Could you check a few things on this drawing? It's one solid part, dimensions in mm from its lowest x, y, z. Round coordinates to 2 decimals unless told otherwise and drop trailing zeros. Write each loop counter-clockwise with the first axis right and the second up, starting at its lowest first coordinate (ties: lowest second). Pieces come first, ordered by that corner, then holes. Notation, with made-up numbers: (36, 42) - (68, 42) arc R20 cw to (68, 67) - close; hole circle Ø2 at (42.5, 0.5). An arc over 180 degrees is marked (long way). Use one line per item in the form item = value. Start each with the question number.
1. Will these pins go through, and if not, where does the flat tip stop? pin 1 (8 mm diameter, centred on x = 4, y = 40, fed in from +Z); pin 2 (6 mm diameter, centred on x = 12.7, y = 31.19, fed in from -Z); pin 3 (5.5 mm diameter, centred on x = 12.7, y = 12.7, fed in from -Z) (1 decimal).
2. I want a section at B-B, the plane y = 12.7. List the corners of the cut face in (x, z) for me (1 decimal).
3. I want a section at A-A, the plane z = 10. List the corners of the cut face in (x, y) for me (1 decimal).
4. We'd pull the mould along Y, two halves only. Please class the marked faces 1, 2, 3 and 4: +Y half, -Y half, draft (parallel to the pull), parting line (faces both ways), or undercut.
5. I want a section at D-D, the plane x = 20.5. List the corners of the cut face in (y, z) for me (1 decimal).
6. If I drill on line 1 along Y through (x, z) = (2, 7.75) (1 decimal); line 2 along Y through (x, z) = (19.25, 4.75) (1 decimal); line 3 along Y through (x, z) = (16.75, 4.75) (1 decimal), over which ranges is the centre line in solid material (lowest first)?
7. I want a section at C-C, the plane y = 40.5. List the corners of the cut face in (x, z) for me (1 decimal).
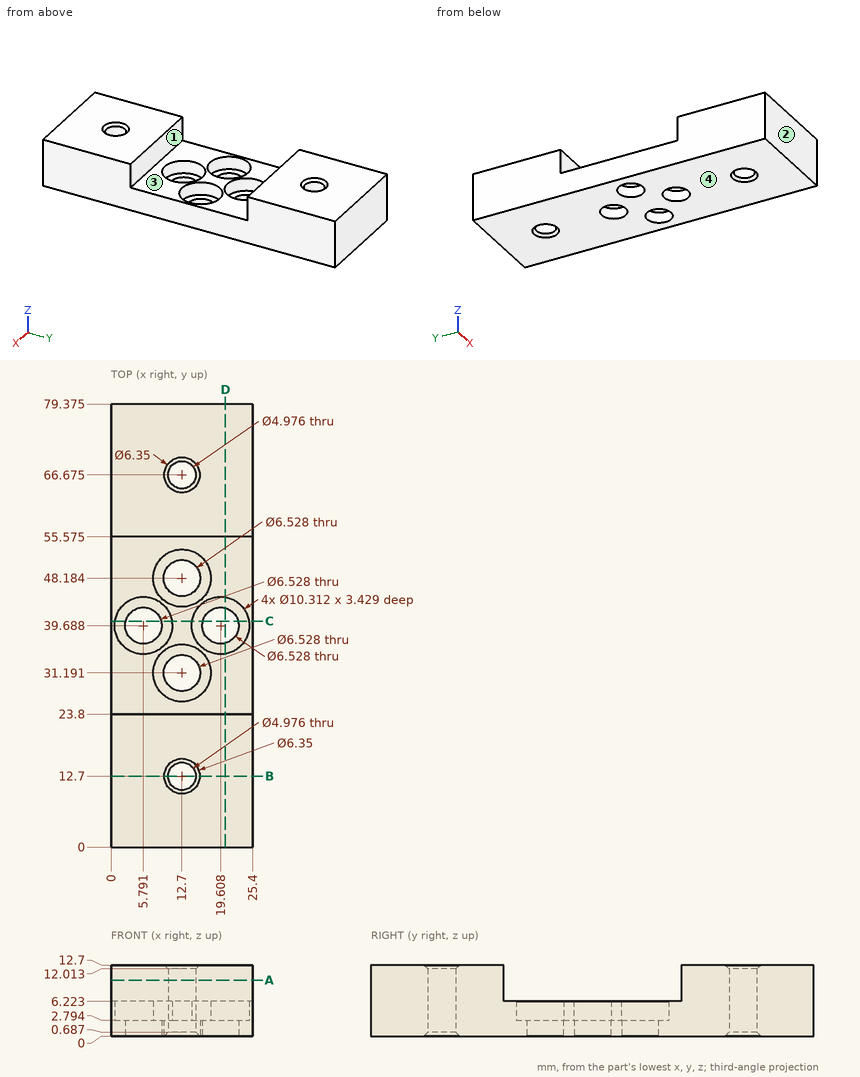
Model answer:
q1.pin_1 = 6.22
q1.pin_2 = through
q1.pin_3 = 0.4
q2.outline = (0, 0) - (9.5, 0) - (10.2, 0.7) - (10.2, 12) - (9.5, 12.7) - (0, 12.7) - close; (15.2, 0.7) - (15.9, 0) - (25.4, 0) - (25.4, 12.7) - (15.9, 12.7) - (15.2, 12) - close
q3.outline = (0, 0) - (25.4, 0) - (25.4, 23.8) - (0, 23.8) - close; (0, 55.6) - (25.4, 55.6) - (25.4, 79.4) - (0, 79.4) - close; hole circle Ø5 at (12.7, 12.7); hole circle Ø5 at (12.7, 66.7)
q4.face_1 = undercut
q4.face_2 = -Y half
q4.face_3 = undercut
q4.face_4 = draft
q5.outline = (0, 0) - (36.5, 0) - (36.5, 2.8) - (34.6, 2.8) - (34.6, 6.2) - (23.8, 6.2) - (23.8, 12.7) - (0, 12.7) - close; (42.8, 0) - (79.4, 0) - (79.4, 12.7) - (55.6, 12.7) - (55.6, 6.2) - (44.8, 6.2) - (44.8, 2.8) - (42.8, 2.8) - close
q6.line_1 = 0 to 23.8, 55.6 to 79.4
q6.line_2 = 0 to 34.5, 44.8 to 79.4
q6.line_3 = 0 to 28, 34.4 to 35.4, 44 to 45, 51.4 to 79.4
q7.outline = (0, 0) - (2.6, 0) - (2.6, 2.8) - (0.7, 2.8) - (0.7, 6.2) - (0, 6.2) - close; (9, 0) - (16.4, 0) - (16.4, 2.8) - (14.5, 2.8) - (14.5, 6.2) - (10.9, 6.2) - (10.9, 2.8) - (9, 2.8) - close; (22.8, 0) - (25.4, 0) - (25.4, 6.2) - (24.7, 6.2) - (24.7, 2.8) - (22.8, 2.8) - close
